Check sheet for the modelled part. Datum: model origin and axes. Units: mm. A direction names the side the tool comes from. Round coordinates to 2 decimals unless told otherwise and drop trailing zeros. Write each loop counter-clockwise with the first axis right and the second up, starting at its lowest first coordinate (ties: lowest second). Pieces come first, ordered by that corner, then holes. Notation, with made-up numbers: (-14.5, 1) - (2.5, 1) arc R27 ccw to (2.5, 34) - close; hole circle Ø3 at (60, -23.75). An arc over 180 degrees is marked (long way). Use one line per item in the form item = value. Start each with the question number.
1) Section check A-A (y = 21). Record the boundary of the cut face in (x, z), then the cut area to 3 significant figures.
2) Section check D-D (z = 10). Record the boundary of the cut face in (x, y), then the cut area to 3 significant figures.
3) Gauge pin test, flat ends, axial feed: P1, Ø1.6, axis at y = 14.5, z = -0.5, coming from the -X side; P2, Ø8, axis at y = 16.5, z = 12.5, coming from the +X side; P3, Ø9.5, axis at y = 21, z = 10.75, coming from the +X side; P4, Ø2, axis at y = 8, z = 6.5, coming from the +X side. Record the tip position at first contact, or that the pin passes through.
4) Draft check along X on faces 6 (the face through (-31, -1.5, 11)), 7 (the face through (-63.414, 16.023, 3.433)), 8 (the face through (-53, 21, -1)). Enter one of: +X half, -X half, draft (parallel to the pull), parting line (faces both ways), or undercut.
5) Section check B-B (x = -7.5). Record the boundary of the cut face in (y, z), then the cut area to 4 significant figures.
6) Scan lines: probe 1 along Z at (x, y) = (-63, 21); probe 2 along Y at (x, z) = (-51.5, 15.5); probe 3 along Z at (x, y) = (-64.8, 21). Record each from-to range of solid material in increasing order.
7) Set-up check for faces 1 (the face through (-28, 6, -1)), 2 (the face through (-37, 21, 21.5)), 3 (the face through (-3, 21, -1)), 4 (the face through (-5, 4, 22)), 5 (the face through (-31.5, 36.3, -1.5)): record each of +Z, -Z, +X, -X, +Y, -Y from which the full face is reachable in a straight line by a thin tool's end or side.
8) Section check C-C (x = -55). Record the boundary of the cut face in (y, z), then the cut area to 4 significant figures.
from build123d import *

# Parameters (mm, degrees)
SALIENTE_EXTRUIR1_DEPTH    = 21.5
SALIENTE_EXTRUIR2_DEPTH    = 1.5
SALIENTE_EXTRUIR3_START    = 1.5
CROQUIS3_W                 = 50
CROQUIS3_H                 = 30
SALIENTE_EXTRUIR3_DEPTH    = 1.5
CORTAR_EXTRUIR1_START      = -1.5
CORTAR_EXTRUIR1_DEPTH      = 1.5
CORTAR_EXTRUIR2_DEPTH      = 1.5
CORTAR_EXTRUIR2_DEPTH_BACK = 3
CROQUIS7_W                 = 21.5
CROQUIS7_H                 = 42
CORTAR_EXTRUIR3_DEPTH      = 10
CORTAR_EXTRUIR3_DEPTH_BACK = 10
CROQUIS8_R                 = 8


with BuildPart() as part:
    # Croquis1 → Saliente-Extruir1 (new body)
    with BuildSketch(Plane.XY):
        with BuildLine():
            Line((-63.5, 43.5), (1.5, 43.5))
            ThreePointArc((1.5, 43.5), (3.220302161, 21), (1.5, -1.5))
            Line((1.5, -1.5), (-63.5, -1.5))
            ThreePointArc((-63.5, -1.5), (-65.220302161, 21), (-63.5, 43.5))
        make_face()
        with BuildLine():
            Line((0, 0), (-62, 0))
            ThreePointArc((-62, 0), (-63.497440295, 21), (-62, 42))
            Line((-62, 42), (0, 42))
            ThreePointArc((0, 42), (1.497440295, 21), (0, 0))
        make_face(mode=Mode.SUBTRACT)
    extrude(amount=SALIENTE_EXTRUIR1_DEPTH)

    # Croquis2 → Saliente-Extruir2 (add)
    with BuildSketch(Plane.XY.offset(21.5)):
        with BuildLine():
            Line((-63.5, 43.5), (1.5, 43.5))
            ThreePointArc((1.5, 43.5), (3.220302161, 21), (1.5, -1.5))
            Line((1.5, -1.5), (-63.5, -1.5))
            ThreePointArc((-63.5, -1.5), (-65.220302161, 21), (-63.5, 43.5))
        make_face()
    extrude(amount=SALIENTE_EXTRUIR2_DEPTH)

    # Croquis3 → Saliente-Extruir3 (add)
    with BuildSketch(Plane(origin=(0, 0, 0), x_dir=(-1, 0, 0), z_dir=(0, 0, -1)).offset(SALIENTE_EXTRUIR3_START)):
        with BuildLine():
            Line((-1.5, 43.5), (63.5, 43.5))
            ThreePointArc((63.5, 43.5), (65.220302161, 21), (63.5, -1.5))
            Line((63.5, -1.5), (-1.5, -1.5))
            ThreePointArc((-1.5, -1.5), (-3.220302161, 21), (-1.5, 43.5))
        make_face()
        with Locations((28, 21)):
            Rectangle(CROQUIS3_W, CROQUIS3_H, mode=Mode.SUBTRACT)
    extrude(amount=-SALIENTE_EXTRUIR3_DEPTH)

    # Croquis4 → Cortar-Extruir1 (cut)
    with BuildSketch(Plane.XY.offset(23).offset(CORTAR_EXTRUIR1_START)):
        with BuildLine():
            Line((-12.279697839, 38), (2.240708907, 38))
            ThreePointArc((2.240708907, 38), (3.220302161, 21), (2.240708907, 4))
            Line((2.240708907, 4), (-12.279697839, 4))
            ThreePointArc((-12.279697839, 4), (-29.279697839, 21), (-12.279697839, 38))
        make_face()
    extrude(amount=CORTAR_EXTRUIR1_DEPTH, mode=Mode.SUBTRACT)

    # Croquis7 → Cortar-Extruir2 (cut, two sides: drawn at the far end of the back side and taken through both)
    with BuildSketch(Plane.ZY.offset(-1.5).offset(-CORTAR_EXTRUIR2_DEPTH_BACK)):
        with Locations((10.75, 21)):
            Rectangle(CROQUIS7_W, CROQUIS7_H)
    extrude(amount=CORTAR_EXTRUIR2_DEPTH + CORTAR_EXTRUIR2_DEPTH_BACK, mode=Mode.SUBTRACT)

    # Croquis8 → Cortar-Extruir3 (cut, two sides: drawn at the far end of the back side and taken through both)
    with BuildSketch(Plane.ZY.offset(63.5).offset(-CORTAR_EXTRUIR3_DEPTH_BACK)):
        with Locations(Location((10.75, 21, 0), (0, 0, 90))):
            Circle(CROQUIS8_R)
    extrude(amount=CORTAR_EXTRUIR3_DEPTH + CORTAR_EXTRUIR3_DEPTH_BACK, mode=Mode.SUBTRACT)


solid = part.part
Results are:
q1.outline = (-65.22, -1.5) - (-53, -1.5) - (-53, 0) - (-63.5, 0) - (-63.5, 2.75) - (-65.22, 2.75) - close; (-65.22, 18.75) - (-63.5, 18.75) - (-63.5, 21.5) - (-29.28, 21.5) - (-29.28, 23) - (-65.22, 23) - close; (-3, -1.5) - (3.22, -1.5) - (3.22, 0) - (-3, 0) - close
q1.area = 91.0 mm²
q2.outline = (-65.01, 13.04) arc R148 ccw to (-63.5, -1.5) - (1.5, -1.5) arc R148 ccw to (1.72, 0) - (-62, 0) arc R148 cw to (-63.28, 13.04) - close; (-65.01, 28.96) - (-63.28, 28.96) arc R148 cw to (-62, 42) - (1.72, 42) arc R148 ccw to (1.5, 43.5) - (-63.5, 43.5) arc R148 ccw to start
q2.area = 241 mm²
q3.P1 = -65.11
q3.P2 = -63.25
q3.P3 = through
q3.P4 = -62.83
q4.face_6 = draft
q4.face_7 = +X half
q4.face_8 = undercut
q5.outline = (-1.5, -1.5) - (6, -1.5) - (6, 0) - (0, 0) - (0, 21.5) - (4, 21.5) - (4, 23) - (-1.5, 23) - close; (36, -1.5) - (43.5, -1.5) - (43.5, 23) - (38, 23) - (38, 21.5) - (42, 21.5) - (42, 0) - (36, 0) - close
q5.area = 103.5 mm²
q6.probe_1 = -1.5 to 0, 21.5 to 23
q6.probe_2 = -1.5 to 0, 42 to 43.5
q6.probe_3 = -1.5 to 2.75, 18.75 to 23
q7.face_1 = -Z
q7.face_2 = +X
q7.face_3 = +Z, -Z
q7.face_4 = +Z, +X
q7.face_5 = -Z, +X, -X, +Y, -Y
q8.outline = (-1.5, -1.5) - (43.5, -1.5) - (43.5, 23) - (-1.5, 23) - close; hole (0, 0) - (42, 0) - (42, 21.5) - (0, 21.5) - close
q8.area = 199.5 mm²
